Autodesk Inventor part; units mm, degrees
ref_plane "Work Plane1" through (0, 8.75, 0) normal (0, 1, 0) x (1, 0, 0)
ref_plane "YZ Plane" through (0, 0, 0) normal (1, 0, 0) x (0, 1, 0)
ref_plane "XZ Plane" through (0, 0, 0) normal (0, 1, 0) x (-1, 0, 0)
sketch "Sketch1" plane through (0, 0, 0) normal (0, 1, 0) x (-1, 0, 0)
  circle A0 centre (0, 0) radius 21
  circle A1 centre (0, 0) radius 4
  dimension "d0" = 42
  dimension "d1" = 8
extrude "Extrusion1" add sketch "Sketch1" along normal blind 10
sketch "Sketch2" plane through (0, 10, 0) normal (0, 1, 0) x (1, 0, 0)
  circle A0 centre (0, 0) radius 4
  circle A1 centre (0, 0) radius 12.5
  dimension "d4" = 8
  dimension "d5" = 25
extrude "Extrusion2" add sketch "Sketch2" along normal blind 6
ref_plane "Work Plane1" through (0, 8.75, 0) normal (0, 1, 0) x (1, 0, 0)
sketch "Sketch3" plane through (0, 8.75, 0) normal (0, 1, 0) x (1, 0, 0)
  circle A0 centre (0, 0) radius 21
  circle A1 centre (0, 0) radius 21
  circle A2 centre (0, 0) radius 20
  dimension "d9" = 1
extrude "Extrusion3" cut sketch "Sketch3" against normal blind 7.5
properties part number "Gt2_60"
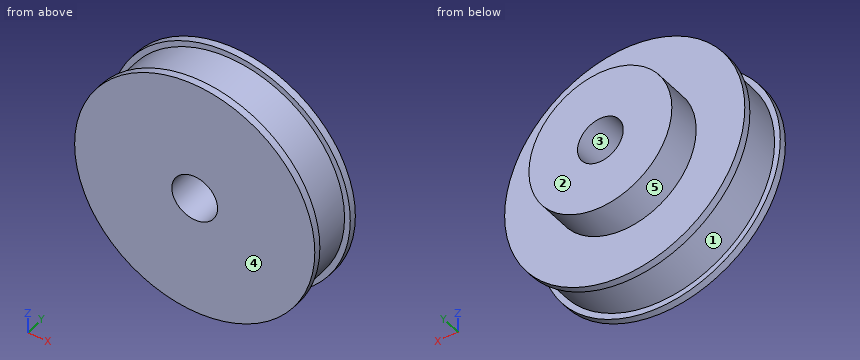
Input: part model. Units: mm. Frame: model coordinates. Face numbers are marked on the shaded views. A direction names the side the tool comes from. Give positions to 0.01 mm unless a question says otherwise; leave off trailing zeros. Loops run counter-clockwise (first coordinate to the right, second up) from the corner with the lowest first, then second, coordinate; pieces in that order, holes last.
1) Section query A-A on y = 3. Return the cut outline in (x, z).
A:
outline: circle Ø40 at (0, 0); hole circle Ø8 at (0, 0)
2) Section query C-C on z = -11.5. Return the cut outline in (x, y), and give its area (3 significant figures).
A:
outline: (-17.57, 0) - (17.57, 0) - (17.57, 1.25) - (16.36, 1.25) - (16.36, 8.75) - (17.57, 8.75) - (17.57, 10) - (4.9, 10) - (4.9, 16) - (-4.9, 16) - (-4.9, 10) - (-17.57, 10) - (-17.57, 8.75) - (-16.36, 8.75) - (-16.36, 1.25) - (-17.57, 1.25) - close
area: 392 mm2
3) Contact query for flat-ended pins moving along their axis: pin 1 (4 mm diameter, centred on y = 14, z = -5, fed in from -X); pin 2 (6 mm diameter, centred on x = -7.5, y = 11.5, fed in from -Z); pin 3 (6.5 mm diameter, centred on x = 0, z = 0, fed in from +Y); pin 4 (2 mm diameter, centred on x = -14.5, y = 3.5, fed in from +Z). Output: stop coordinate, or through.
A:
pin 1: stops at x = -12.13
pin 2: stops at z = -20.42
pin 3: passes through
pin 4: stops at z = 14.76
4) Line query: L1, parallel to X at y = 10.5, z = 0; L2, parallel to X at y = 5, z = 0. Output: solid intervals per line, ascending.
A:
L1: x = -12.5 to -4, 4 to 12.5
L2: x = -20 to -4, 4 to 20
5) Mould query, pull axis Y, two halves, no side actions, for the marked faces 1, 2 and 3. Classes: released by +Y, released by -Y, zero draft, split by the parting line, or undercut.
A:
face 1: undercut
face 2: released by +Y
face 3: zero draft
6) Section query D-D on x = 14.5. Return the cut outline in (y, z), and give its area (3 significant figures).
A:
outline: (0, -15.19) - (1.25, -15.19) - (1.25, -13.77) - (8.75, -13.77) - (8.75, -15.19) - (10, -15.19) - (10, 15.19) - (8.75, 15.19) - (8.75, 13.77) - (1.25, 13.77) - (1.25, 15.19) - (0, 15.19) - close
area: 283 mm2
7) Reachability of the marked faces 4 and 5 from +Z, -Z, +X, -X, +Y, -Y: full face, straight path, thin tool, end or side. Return the list, or none.
A:
face 4: +Z, -Z, +X, -X, -Y
face 5: +Y
